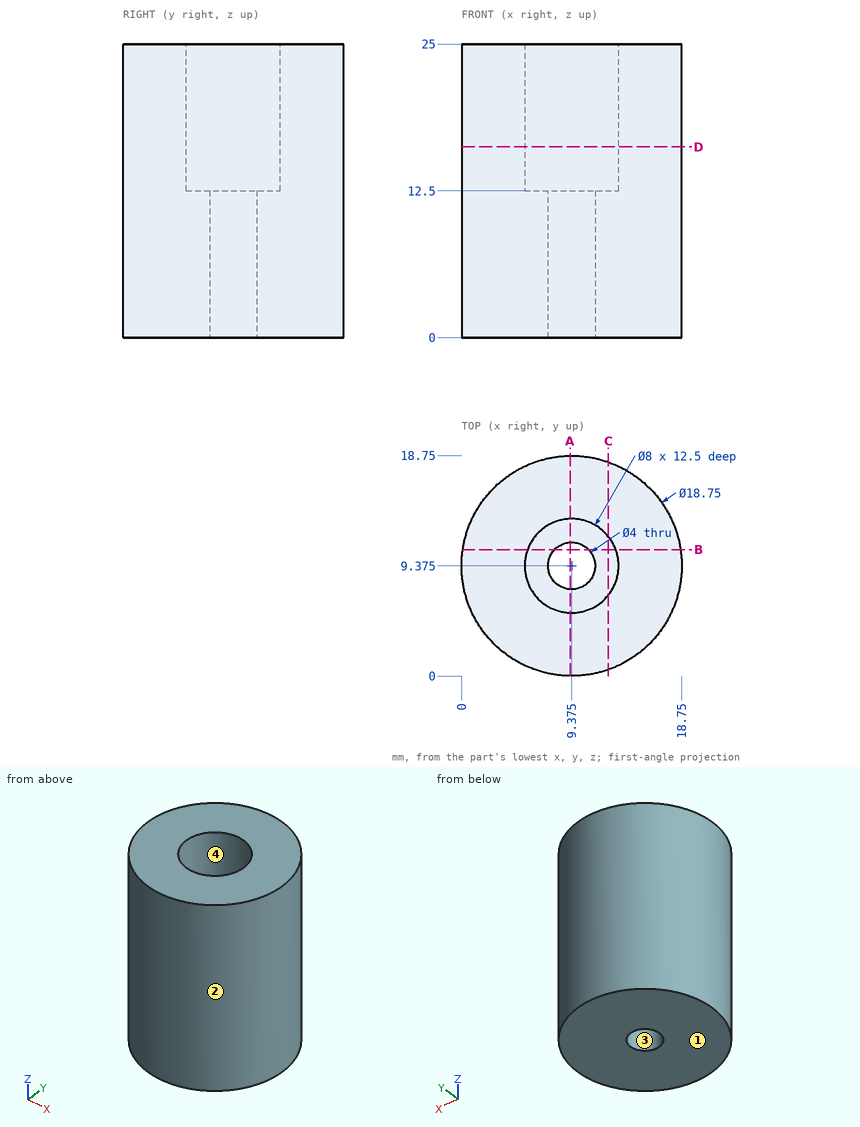
Answer from the drawing. Dimensions are ordinates in mm from the lowest x, y and z of the part. Coordinates: 2 decimals unless noted, no trailing zeros. Write each loop counter-clockwise with the first axis right and the second up, starting at its lowest first coordinate (ties: lowest second). Pieces come first, ordered by that corner, then holes. Notation, with made-up numbers: M -22.75,16 L 25.25,16 A15 cw 25.25,41 Z; hole C 18,-15.5 d2. An arc over 180 degrees is marked long. Use one line per item in the form item = value. Start each with the question number.
1. Straight lines are drawn through the part: probe 1 along Z at (x, y) = (9.5, 12); probe 2 along X at (y, z) = (11, 10.5); probe 3 along X at (y, z) = (9.75, 6). For each, find the intervals that lie inside material, in ascending order. Write a range as from..to.
2. The part is cut by section A-A (x = 9.25). Give the vertices of the cut face in (y, z).
3. The mould has two halves that part along X. Classify the marked faces 1, 2, 3 and 4: released by +X, released by -X, zero draft, split by the parting line, or undercut.
4. The part is cut by section C-C (x = 12.5). Give the vertices of the cut face in (y, z), plus the area to 3 significant figures.
5. The part is cut by section D-D (z = 16.25). Give the vertices of the cut face in (x, y) (3 decimals).
6. Each of these flat-tipped pins is pushed along its axis until it touches: P1, Ø4, axis at x = 6, z = 18.5, coming from the -Y side; P2, Ø1.5, axis at y = 16.5, z = 8, coming from the +X side; P3, Ø2, axis at y = 16.5, z = 12.5, coming from the -X side. Where does it stop, or does it pass through?
7. The part is cut by section B-B (y = 10.75). Give the vertices of the cut face in (x, z).
Evaluation:
q1.probe_1 = 0..12.5
q1.probe_2 = 0.14..8.21, 10.54..18.61
q1.probe_3 = 0.01..7.41, 11.34..18.74
q2.outline = M 0,0 L 7.38,0 L 7.38,12.5 L 5.38,12.5 L 5.38,25 L 0,25 Z; M 11.37,0 L 18.75,0 L 18.75,25 L 13.37,25 L 13.37,12.5 L 11.37,12.5 Z
q3.face_1 = zero draft
q3.face_2 = split by the parting line
q3.face_3 = undercut
q3.face_4 = undercut
q4.outline = M 0.54,0 L 18.21,0 L 18.21,25 L 11.87,25 L 11.87,12.5 L 6.88,12.5 L 6.88,25 L 0.54,25 Z
q4.area = 380 mm^2
q5.outline = C 9.375,9.375 d18.75; hole C 9.375,9.375 d8
q6.P1 = 0.1
q6.P2 = 16.25
q6.P3 = 2.28
q7.outline = M 0.1,0 L 7.92,0 L 7.92,12.5 L 5.62,12.5 L 5.62,25 L 0.1,25 Z; M 10.83,0 L 18.65,0 L 18.65,25 L 13.13,25 L 13.13,12.5 L 10.83,12.5 Z
